Autodesk Inventor part; units mm, degrees
ref_plane "YZ Plane" through (0, 0, 0) normal (1, 0, 0) x (0, 1, 0)
ref_plane "XZ Plane" through (0, 0, 0) normal (0, 1, 0) x (-1, 0, 0)
ref_plane "XY Plane" through (0, 0, 0) normal (0, 0, 1) x (1, 0, 0)
sketch "Skizze1" plane through (0, 0, 0) normal (0, 0, 1) x (1, 0, 0)
  line L0 (-3157.2887, 244.4054) -> (-1410.3053, 244.4054)
  line L1 (-1410.3053, 199.2768) -> (-1410.3053, 244.4054)
  arc A0 (-1520.1704, 149.4054) -> (-1410.3053, 199.2768) centre (-1628.683, 534.4054) ccw
  line L2 (-3054.6765, 149.4054) -> (-1520.1704, 149.4054)
  arc A1 (-3157.2887, 244.4054) -> (-3054.6765, 149.4054) centre (-2978.683, 334.4054) ccw
  point P0 (-2370.1189, 0)
  point P1 (-1410.3053, 199.2768)
  point P2 (-1410.3053, 244.4054)
  dimension "d59" = 400
  dimension "d60" = 200
  dimension "d61" = 95
  dimension "d62" = 0
  dimension "d63" = 0
  dimension "d64" = 45.1286
  dimension "d65" = 0
  dimension "d66" = 45.1286
  dimension "d67" = 109.865
  dimension "d68" = 109.865
  dimension "d69" = 95
  dimension "d70" = 959.8136
  dimension "d71" = 244.4054
  dimension "d72" = 1568.3777
  dimension "d73" = 90
  dimension "d74" = 1644.3711
  dimension "d75" = 1644.3711
  dimension "d76" = 1746.9834
  dimension "d77" = 1746.9834
extrude "Extrusion1" add sketch "Skizze1" along normal blind 20
sketch "Skizze2" plane through (-3157.2887, 244.4054, 0) normal (0, 1, 0) x (1, 0, 0)
  line L0 (1746.9834, -20) -> (1856.261, -20)
  ellipse E0 centre (1857.974, 0) end of major axis (1731.8988, 18.1709) minor radius 65.6716 (1734.0318, 0) -> (1746.9834, -20) ccw
  line L1 (1746.9834, 0) -> (0, 0)
  line L2 (1746.9834, 0) -> (1746.9834, -20)
  line L3 (1856.261, -20) -> (1856.261, 0)
  line L4 (1856.261, 0) -> (1734.0318, 0)
  line L5 (1637.1184, 0) -> (1746.9834, 0)
  point P0 (3157.2887, 0)
  point P1 (1734.0318, 0)
  dimension "d59" = 400
  dimension "d87" = 0
  dimension "d88" = 109.2776
extrude "Extrusion2" cut sketch "Skizze2" against normal through all
properties part number "HolzLatteRechts"
Geometry check sheet. Reference: the model listing, model coordinates, mm. Coordinates: 2 decimals unless noted, no trailing zeros. Loops run counter-clockwise (first coordinate to the right, second up) from the corner with the lowest first, then second, coordinate; pieces in that order, holes last.
Item 1: Sectioned sample at A-A, the plane y = 175. Record the boundary of the cut face in (x, z).
Item 2: Go/stop test with flat-tipped pins: pin 1 Ø2 at (y, z) = (211.5, 7.5) entering from +X; pin 2 Ø1 at (y, z) = (188.5, 2.5) entering from +X; pin 3 Ø12 at (y, z) = (224.5, 3.5) entering from +X. Record where each tip stops, or that it passes through.
Item 3: Thickness scan on line 1 (X direction, y = 195, z = 15.5); line 2 (X direction, y = 237, z = 13.75). Record the ranges inside material, lowest first.
Check result:
1. outline: (-3099.47, 0) - (-1453.1, 0) - (-1453.1, 20) - (-3099.47, 20) - close
2. pin 1: stops at x = -1419.13
2. pin 2: stops at x = -1426.95
2. pin 3: stops at x = -1418.52
3. line 1: x = -3122.09 to -1417.01
3. line 2: x = -3153.36 to -1415.58
